Autodesk Inventor part; units mm, degrees
ref_plane "Work Plane1" through (0, 38.1, 5.08) normal (0, 1, 0) x (-1, 0, 0)
ref_plane "YZ Plane" through (0, 0, 0) normal (1, 0, 0) x (0, 1, 0)
ref_plane "XZ Plane" through (0, 0, 0) normal (0, 1, 0) x (-1, 0, 0)
sketch "Sketch1" plane through (0, 0, 0) normal (0, 0, 1) x (1, 0, 0)
  line L0 (0, 0) -> (0, 76.2)
  line L1 (0, 76.2) -> (-10.16, 76.2)
  line L2 (-10.16, 76.2) -> (-10.16, 63.5)
  line L3 (-10.16, 63.5) -> (-24.13, 46.99)
  line L4 (-24.13, 46.99) -> (-31.75, 46.99)
  line L5 (-31.75, 46.99) -> (-31.75, 40.64)
  line L6 (-21.59, 35.56) -> (-31.75, 35.56)
  line L7 (-31.75, 35.56) -> (-31.75, 29.21)
  line L8 (-31.75, 29.21) -> (-24.13, 29.21)
  line L9 (-24.13, 29.21) -> (-10.16, 12.7)
  line L10 (-10.16, 12.7) -> (-10.16, 0)
  line L11 (-10.16, 0) -> (0, 0)
  line L12 (-31.75, 40.64) -> (-21.59, 40.64)
  line L13 (-21.59, 40.64) -> (-21.59, 35.56)
  line L14 (-21.59, 38.1) -> (-22.098, 38.1) construction
  dimension "d1" = 10.16
  dimension "d2" = 31.75
  dimension "d3" = 76.2
  dimension "d5" = 7.62
  dimension "d8" = 5.08
  dimension "d11" = 38.1
  dimension "d12" = 6.35
  dimension "d14" = 12.7
  dimension "d23" = 10.16
extrude "Extrusion1" add sketch "Sketch1" along normal blind 5.08
fillet "Fillet1" radius 3.175 4 edges at (-10.16, 12.7, 2.54) (-24.13, 29.21, 2.54) (-10.16, 63.5, 2.54) (-24.13, 46.99, 2.54)
sketch "Sketch2" plane through (0, 0, 5.08) normal (0, 0, 1) x (1, 0, 0)
  line L0 (-10.16, 11.537) -> (-10.16, 0)
  line L1 (-10.16, 0) -> (0, 0)
  line L2 (0, 0) -> (0, 76.2)
  line L3 (0, 76.2) -> (-10.16, 76.2)
  line L4 (-10.16, 76.2) -> (-10.16, 64.663)
  line L5 (-10.9112, 62.6122) -> (-23.1788, 48.1141)
  line L6 (-25.6026, 46.99) -> (-31.75, 46.99)
  line L7 (-31.75, 46.99) -> (-31.75, 40.64)
  line L8 (-31.75, 40.64) -> (-21.59, 40.64)
  line L9 (-21.59, 40.64) -> (-21.59, 35.56)
  line L10 (-21.59, 35.56) -> (-31.75, 35.56)
  line L11 (-31.75, 35.56) -> (-31.75, 29.21)
  line L12 (-31.75, 29.21) -> (-25.6026, 29.21)
  line L13 (-23.1788, 28.0859) -> (-10.9112, 13.5878)
  line L14 (-24.13, 46.99) -> (-31.75, 46.99) construction
  line L15 (-27.94, 46.99) -> (-27.94, 40.64) construction
  line L16 (-31.75, 40.64) -> (-21.59, 40.64) construction
  line L17 (-29.4005, 46.99) -> (-29.4005, 40.64)
  line L18 (-26.4795, 46.99) -> (-26.4795, 40.64)
  line L19 (0, 0) -> (0, 76.2) construction
  line L20 (0, 38.1) -> (-22.098, 38.1) construction
  line L21 (-29.4005, 29.21) -> (-29.4005, 35.56)
  line L22 (-26.4795, 29.21) -> (-26.4795, 35.56)
  line L23 (-10.16, 12.7) -> (-10.16, 0)
  line L24 (-10.16, 5.08) -> (0, 5.08)
  line L25 (-10.16, 8.001) -> (0, 8.001)
  line L26 (-10.16, 71.12) -> (0, 71.12)
  line L27 (-10.16, 68.199) -> (0, 68.199)
  arc A0 (-23.1788, 28.0859) -> (-25.6026, 29.21) centre (-25.6026, 26.035) ccw
  arc A1 (-10.16, 11.537) -> (-10.9112, 13.5878) centre (-13.335, 11.537) ccw
  arc A2 (-10.9112, 62.6122) -> (-10.16, 64.663) centre (-13.335, 64.663) ccw
  arc A3 (-25.6026, 46.99) -> (-23.1788, 48.1141) centre (-25.6026, 50.165) ccw
  dimension "d18" = 1.4605
  dimension "d19" = 1.4605
  dimension "d21" = 2.921
  dimension "d22" = 5.08
sketch "Sketch3" plane through (-31.75, 46.99, 0) normal (0, 1, 0) x (1, 0, 0)
  line L0 (3.81, -5.08) -> (3.81, 0) construction
  circle A0 centre (3.81, -2.54) radius 1.4605
  point P0 (31.75, 0)
  dimension "d24" = 2.921
extrude "Extrusion2" cut sketch "Sketch3" against normal blind 25.4
sketch "Sketch4" plane through (-10.16, 0, 0) normal (-1, 0, 0) x (0, 0, 1)
  line L0 (0, 0) -> (0, 76.2) construction
  line L1 (0, 12.7) -> (0, 0) construction
  line L2 (0, 6.5405) -> (5.08, 6.5405) construction
  line L3 (0, 0) -> (5.08, 0) construction
  circle A0 centre (2.54, 6.5405) radius 1.4605
  point P0 (5.08, 5.08)
  dimension "d27" = 6.5405
  dimension "d28" = 2.921
extrude "Extrusion3" cut sketch "Sketch4" against normal blind 25.4
ref_plane "Work Plane1" through (0, 38.1, 5.08) normal (0, 1, 0) x (-1, 0, 0)
mirror "Mirror1" about plane through (0, 38.1, 5.08) normal (0, 1, 0) of "Extrusion3"
equation "\"d19\" = d18"
properties part number "mount 3D print"
Geometry: final body of the model. Coordinates: model frame, mm. A direction names the side the tool comes from. Round coordinates to 2 decimals unless told otherwise and drop trailing zeros. Order: outer loops, then holes, each group sorted by start corner. A loop starts at its lowest first (then second) coordinate and runs counter-clockwise, first axis right, second up. Notation, with made-up numbers: M -22.5,-11.75 L -10.5,-11.75 A21 cw -10.5,14.25 Z; hole C 18.5,77 d6. An arc over 180 degrees is marked long. Use one line per item in the form item = value. Start each with the question number.
Q1. Access query for faces 4 (the face through (-26, 40.64, 3)), 5 (the face through (-5, 76.2, 3)). Directions: +Z, -Z, +X, -X, +Y, -Y. A direction counts if a zero-diameter tool reaches every point of the face in a straight line with its end or side. Return the directions, or none.
Q2. Pin query (flat end, axial travel): pin 1 Ø1.8 at (x, z) = (-27.94, 2.54) entering from -Y; pin 2 Ø1.5 at (y, z) = (38.5, 3) entering from -X; pin 3 Ø1 at (y, z) = (55, 2.5) entering from -X; pin 4 Ø2.5 at (x, z) = (-28, 2) entering from -Y. Return the tip coordinate at first contact, or that it passes through.
Q3. Material intervals for line 1 (Y direction, x = -4.5, z = 2.54); line 2 (X direction, y = 33.25, z = 2.54); line 3 (Z direction, x = -27.94, y = 31.25), sorted ascending. Write a range as [from, to].
Q4. Cut plane D-D (x = -19). Return loops of the section in (y, z), and give its area (3 significant figures).
Q5. Cut plane C-C (y = 54). Return loops of the section in (x, z), and give its area (3 significant figures).
Q6. Mould query, pull axis X, two halves, no side actions, for faces 1 (the face through (-30, 46.99, 3)), 2 (the face through (-16.959, 55.465, 2.504)), 3 (the face through (-29.016, 43.859, 1.553)). Classes: +X half, -X half, draft (parallel to the pull), parting line (faces both ways), or undercut.
Q7. Cut plane A-A (z = 2.54). Count the separate pieces of the cut face and the enclosed holes in it, and give its area (3 significant figures).
Q8. Cut plane B-B (x = -27.94). Return loops of the section in (y, z).
Geometry results:
q1.face_4 = +Z, -Z, -X
q1.face_5 = +Z, -Z, +X, -X, +Y
q2.pin_1 = through
q2.pin_2 = -21.59
q2.pin_3 = -17.78
q2.pin_4 = 29.21
q3.line_1 = [0, 5.08], [8, 68.2], [71.12, 76.2]
q3.line_2 = [-31.75, -29.4], [-26.48, 0]
q3.line_3 = [0, 1.08], [4, 5.08]
q4.outline = M 23.15,0 L 53.05,0 L 53.05,5.08 L 23.15,5.08 Z
q4.area = 152 mm^2
q5.outline = M -18.2,0 L 0,0 L 0,5.08 L -18.2,5.08 Z
q5.area = 92.4 mm^2
q6.face_1 = draft
q6.face_2 = -X half
q6.face_3 = undercut
q7.separate_pieces = 5
q7.enclosed_holes = 0
q7.area = 1,240 mm^2
q8.outline = M 29.21,0 L 35.56,0 L 35.56,1.08 L 29.21,1.08 Z; M 29.21,4 L 35.56,4 L 35.56,5.08 L 29.21,5.08 Z; M 40.64,0 L 46.99,0 L 46.99,1.08 L 40.64,1.08 Z; M 40.64,4 L 46.99,4 L 46.99,5.08 L 40.64,5.08 Z
